Source: CAD feature listing. Evaluate the final solid. Frame: model axes, mm. Face numbers are marked on the shaded views. A direction names the side the tool comes from. Give positions to 0.01 mm unless a question says otherwise; leave off trailing zeros. Loops run counter-clockwise (first coordinate to the right, second up) from the corner with the lowest first, then second, coordinate; pieces in that order, holes last. Notation, with made-up numbers: M 20.5,22 L 31.5,22 A9 cw 31.5,35 Z; hole C 21,18 d1. An arc over 180 degrees is marked long. Answer in a Markdown table with one row per item.
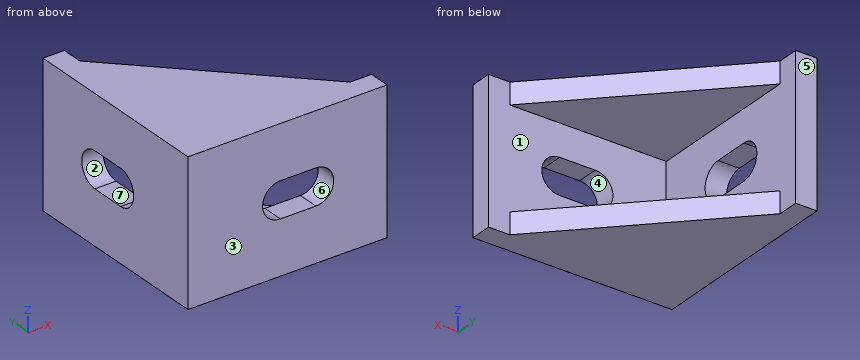
```python
from build123d import *

# Parameters (mm, degrees)
BOSS_EXTRUDE1_DEPTH = 20
CUT_EXTRUDE1_DEPTH  = 14
CUT_EXTRUDE2_DEPTH  = 14
CUT_EXTRUDE3_DEPTH  = 14


with BuildPart() as part:
    # Sketch1 → Boss-Extrude1 (new body)
    with BuildSketch(Plane.XY):
        Polygon((0, 0), (0, 28), (3, 28), (3, 25), (25, 3), (28, 3), (28, 0), align=None)
    extrude(amount=-BOSS_EXTRUDE1_DEPTH)

    # Sketch2 → Cut-Extrude1 (cut)
    with BuildSketch(Plane.XY.offset(-3)):
        Polygon((3, 25), (3, 3), (25, 3), align=None)
    extrude(amount=-CUT_EXTRUDE1_DEPTH, mode=Mode.SUBTRACT)

    # Sketch3 → Cut-Extrude2 (cut)
    with BuildSketch(Plane(origin=(0, 3, 0), x_dir=(1, 0, 0), z_dir=(0, 1, 0))):
        with BuildLine():
            Line((18, 7.5), (13, 7.5))
            ThreePointArc((13, 7.5), (10.5, 10), (13, 12.5))
            Line((13, 12.5), (18, 12.5))
            ThreePointArc((18, 12.5), (20.5, 10), (18, 7.5))
        make_face()
    extrude(amount=-CUT_EXTRUDE2_DEPTH, mode=Mode.SUBTRACT)

    # Sketch4 → Cut-Extrude3 (cut)
    with BuildSketch(Plane(origin=(3, 0, 0), x_dir=(0, 0, -1), z_dir=(1, 0, 0))):
        with BuildLine():
            Line((7.5, 13), (7.5, 18))
            ThreePointArc((7.5, 18), (10, 20.5), (12.5, 18))
            Line((12.5, 18), (12.5, 13))
            ThreePointArc((12.5, 13), (10, 10.5), (7.5, 13))
        make_face()
    extrude(amount=-CUT_EXTRUDE3_DEPTH, mode=Mode.SUBTRACT)


solid = part.part
```
1) Material intervals for L1, parallel to Z at x = 19.25, y = 3.25; L2, parallel to Y at x = 18.75, z = -14; L3, parallel to Z at x = 2, y = 13.75, sorted ascending.
Reply:
| item | result |
|---|---|
| L1 | z = -20 to -17, -3 to 0 |
| L2 | y = 0 to 3 |
| L3 | z = -20 to -12.5, -7.5 to 0 |
2) Pull-direction query (Y, two-part tool) for the marked faces 5, 6 and 7; classes: released by +Y, released by -Y, zero draft, split by the parting line, or undercut.
Reply:
| item | result |
|---|---|
| face 5 | released by +Y |
| face 6 | zero draft |
| face 7 | undercut |
3) Section C-C, the plane y = 4.75. Return loops of the section in (x, z).
Reply:
| item | result |
|---|---|
| outline | M 0,-20 L 23.25,-20 L 23.25,-17 L 3,-17 L 3,-3 L 23.25,-3 L 23.25,0 L 0,0 Z |
4) Pin query (flat end, axial travel): pin 1 Ø1.5 at (y, z) = (21.5, -9.5) entering from +X; pin 2 Ø6 at (x, z) = (20, -11.5) entering from +Y. Return the tip coordinate at first contact, or that it passes through.
Reply:
| item | result |
|---|---|
| pin 1 | stops at x = 3 |
| pin 2 | stops at y = 3 |
5) Set-up query: the marked faces 1, 2, 3 and 4. Return all of +Z, -Z, +X, -X, +Y, -Y with unobstructed straight access to the full face (end or side cutting, diameter ignored); none if empty.
Reply:
| item | result |
|---|---|
| face 1 | +X, +Y |
| face 2 | +X, -X |
| face 3 | +Z, -Z, +X, -X, -Y |
| face 4 | +Y, -Y |
6) Section D-D, the plane x = 8. Return loops of the section in (y, z), then the cut area to 3 significant figures.
Reply:
| item | result |
|---|---|
| outline | M 0,-20 L 20,-20 L 20,-17 L 3,-17 L 3,-3 L 20,-3 L 20,0 L 0,0 Z |
| area | 162 mm² |
7) Section A-A, the plane z = -10. Return loops of the section in (x, y), then the cut area to 3 significant figures.
Reply:
| item | result |
|---|---|
| outline | M 0,0 L 10.5,0 L 10.5,3 L 3,3 L 3,10.5 L 0,10.5 Z; M 0,20.5 L 3,20.5 L 3,28 L 0,28 Z; M 20.5,0 L 28,0 L 28,3 L 20.5,3 Z |
| area | 99.0 mm² |
8) Section B-B, the plane x = 15.5. Return loops of the section in (y, z).
Reply:
| item | result |
|---|---|
| outline | M 0,-20 L 12.5,-20 L 12.5,-17 L 3,-17 L 3,-12.5 L 0,-12.5 Z; M 0,-7.5 L 3,-7.5 L 3,-3 L 12.5,-3 L 12.5,0 L 0,0 Z |
